Verification items for the finished model (mm, model axes). Give positions to 0.01 mm unless a question says otherwise; leave off trailing zeros. Loops run counter-clockwise (first coordinate to the right, second up) from the corner with the lowest first, then second, coordinate; pieces in that order, holes last. Notation, with made-up numbers: M -8,-5 L 4,-5 A15 cw 4,23 Z; hole C -35.5,45 d11. An arc over 180 degrees is marked long. Use a Markdown table: item, result.
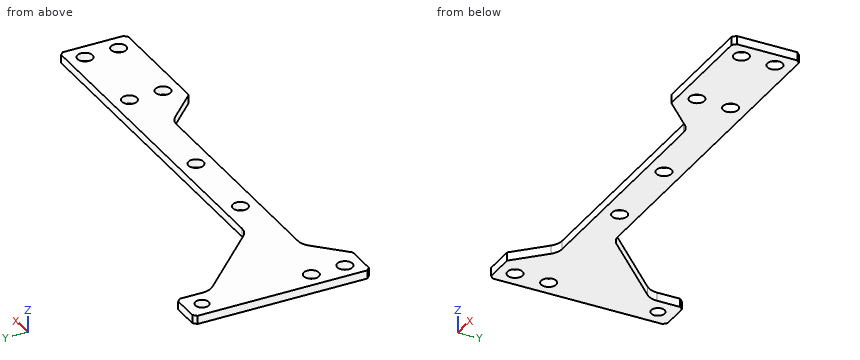
from build123d import *

# Parameters (mm, degrees)
SKETCH_1_R          = 4.5
SKETCH_1_R_2        = 4
EXTRUDE_1_DEPTH     = 5
CHAMFER_2_SIZE      = 20
CHAMFER_3_SIZE      = 20
SKETCH_2_R          = 4.5
CUT_EXTRUDE_1_DEPTH = 5
FILLET_1_R          = 10
CHAMFER_4_SIZE      = 2
SKETCH_3_R          = 4.5
CUT_EXTRUDE_2_DEPTH = 10


with BuildPart() as part:
    # 草图1 → 凸台-拉伸1 (new body)
    with BuildSketch(Plane.XY):
        Polygon((-215, 70), (-215, 75), (-215, 95), (-195, 95), (-195, 75), (-150, 30), (60, 30), (60, 10), (60, -10), (40, -10), (10, -10), (-10, -10), (-10, 10), (-195, 10), (-195, -10), (-215, -10), (-215, 10), align=None)
        Circle(SKETCH_1_R, mode=Mode.SUBTRACT)
        with Locations((50, 0)):
            Circle(SKETCH_1_R, mode=Mode.SUBTRACT)
        with Locations((-205, 20)):
            Circle(SKETCH_1_R, mode=Mode.SUBTRACT)
        with Locations((0, 20)):
            Circle(SKETCH_1_R, mode=Mode.SUBTRACT)
        with Locations((-205, 0)):
            Circle(SKETCH_1_R, mode=Mode.SUBTRACT)
        with Locations((-205, 85)):
            Circle(SKETCH_1_R_2, mode=Mode.SUBTRACT)
    extrude(amount=EXTRUDE_1_DEPTH)

    # 倒角2
    chamfer_2_edges = [part.edges().sort_by_distance(p)[0] for p in [
        (-10, 10, 2.5),
    ]]
    chamfer(chamfer_2_edges, length=CHAMFER_2_SIZE - 0.0001)  # a hair under: the kernel refuses the full size

    # 倒角3
    chamfer_3_edges = [part.edges().sort_by_distance(p)[0] for p in [
        (-195, 10, 2.5),
    ]]
    chamfer(chamfer_3_edges, length=CHAMFER_3_SIZE - 0.0001)  # a hair under: the kernel refuses the full size

    # 草图2 → 切除-拉伸1 (cut)
    with BuildSketch(Plane.XY.offset(5)):
        with Locations((-125, 19.986)):
            Circle(SKETCH_2_R)
        with Locations((-75, 19.986)):
            Circle(SKETCH_2_R)
    extrude(amount=-CUT_EXTRUDE_1_DEPTH, mode=Mode.SUBTRACT)

    # 圆角1
    fillet_1_edges = [part.edges().sort_by_distance(p)[0] for p in [
        (-195, 75, 2.5),
        (-150, 30, 2.5),
        (-29.9999, 10, 2.5),
        (-175.0001, 10, 2.5),
    ]]
    fillet(fillet_1_edges, radius=FILLET_1_R)

    # 倒角4
    chamfer_4_edges = [part.edges().sort_by_distance(p)[0] for p in [
        (60, 30, 2.5),
        (60, -10, 2.5),
        (-215, -10, 2.5),
        (-215, 95, 2.5),
        (-195, 95, 2.5),
    ]]
    chamfer(chamfer_4_edges, length=CHAMFER_4_SIZE)

    # 草图3 → 切除-拉伸2 (cut)
    with BuildSketch(Plane.XY.offset(5)):
        with Locations((50, 20)):
            Circle(SKETCH_3_R)
    extrude(amount=-CUT_EXTRUDE_2_DEPTH, mode=Mode.SUBTRACT)


solid = part.part
(1) Material ranges on line 1 (Y direction, x = -205, z = 1.5); line 2 (Y direction, x = 0, z = 3.45); line 3 (Y direction, x = -103, z = 0.25), recorded low to high.
Results below:
| item | result |
|---|---|
| line 1 | -10 to -4.5, 4.5 to 15.5, 24.5 to 81, 89 to 95 |
| line 2 | -10 to -4.5, 4.5 to 15.5, 24.5 to 30 |
| line 3 | 10 to 30 |
(2) Cross-section at B-B on y = 0. Record the cut outline in (x, z), then the cut area to 3 significant figures.
Results below:
| item | result |
|---|---|
| outline | M -215,0 L -209.5,0 L -209.5,5 L -215,5 Z; M -200.5,0 L -185,0 L -185,5 L -200.5,5 Z; M -20,0 L -4.5,0 L -4.5,5 L -20,5 Z; M 4.5,0 L 45.5,0 L 45.5,5 L 4.5,5 Z; M 54.5,0 L 60,0 L 60,5 L 54.5,5 Z |
| area | 415 mm^2 |
(3) Cross-section at D-D on z = 1.85. State how many separate pieces and enclosed holes the cut face has, then the cut area to 3 significant figures.
Results below:
| item | result |
|---|---|
| separate pieces | 1 |
| enclosed holes | 9 |
| area | 9,450 mm^2 |
(4) Cross-section at A-A on x = -205. Record the cut outline in (y, z).
Results below:
| item | result |
|---|---|
| outline | M -10,0 L -4.5,0 L -4.5,5 L -10,5 Z; M 4.5,0 L 15.5,0 L 15.5,5 L 4.5,5 Z; M 24.5,0 L 81,0 L 81,5 L 24.5,5 Z; M 89,0 L 95,0 L 95,5 L 89,5 Z |
(5) Cross-section at C-C on x = 50. Record the cut outline in (y, z).
Results below:
| item | result |
|---|---|
| outline | M -10,0 L -4.5,0 L -4.5,5 L -10,5 Z; M 4.5,0 L 15.5,0 L 15.5,5 L 4.5,5 Z; M 24.5,0 L 30,0 L 30,5 L 24.5,5 Z |
(6) Gauge pin test, flat ends, axial feed: P1, Ø3, axis at y = 62.5, z = 1, coming from the +X side; P2, Ø2.5, axis at x = -78, z = 2, coming from the -Y side; P3, Ø1, axis at x = -164, z = 3, coming from the +Y side. Record the tip position at first contact, or that the pin passes through.
Results below:
| item | result |
|---|---|
| P1 | x = -181 |
| P2 | y = 10 |
| P3 | y = 44.5 |
